```python
from build123d import *

# Parameters (mm, degrees)
F1_DEPTH = 76.2
F3_ANGLE = 90
F4_DEPTH = 203.2


with BuildPart() as f1:
    # F0 (on Front) → F1 (new body)
    with BuildSketch(Plane.XZ):
        Polygon((-6.5709403187, 0), (-3.175, -5.2222484378), (3.175, -5.2222484378), (6.7875643598, 0), (3.175, 5.2222484378), (-3.175, 5.2222484378), align=None)
    extrude(amount=F1_DEPTH)

    # F2 (on Front) → F3 (revolve)
    with BuildSketch(Plane.XZ):
        Polygon((-3.175, -5.2600912928), (3.175, -5.2600912928), (6.8761393004, 0), (3.175, 5.2600912928), (-3.175, 5.2600912928), (-6.7797889493, 0), align=None)
    revolve(axis=Axis((0, 0, 5.2600912928), (1, 0, 0)), revolution_arc=F3_ANGLE)

    # F4 (add): a face of the model
    f4_faces = [f1.faces().sort_by_distance(p)[0] for p in [
        (0.0270197551, 5.2600912928, 5.2600912928),
    ]]
    extrude(f4_faces, amount=F4_DEPTH)


solid = f1.part
```
Work out the finished part from the listing and answer in its coordinate system (mm). A direction names the side the tool comes from. Coordinates: 2 decimals unless noted, no trailing zeros. Write each loop counter-clockwise with the first axis right and the second up, starting at its lowest first coordinate (ties: lowest second). Pieces come first, ordered by that corner, then holes.
Q1. Each of these flat-tipped pins is pushed along its axis until it touches: pin 1 Ø7 at (x, y) = (0.5, -37) entering from -Z; pin 2 Ø1.5 at (x, z) = (-5, 157) entering from +Y; pin 3 Ø7 at (x, y) = (0.5, -51) entering from +Z. Where does it stop, or does it pass through?
Q2. A cutting plane is placed at B-B, the plane z = 184. Give the vertices of the cut face in (x, y) (3 decimals).
Q3. Which of the six approach directions +Z, -Z, +X, -X, +Y, -Y give full straight-line access (tool end or side, diameter ignored) to faces 1 (the face through (-4.95, 2.59, 105.44)), 2 (the face through (0, -38, 5.222)), 3 (the face through (5.051, 2.667, 105.438))?
Q4. A cutting plane is placed at C-C, the plane y = -60. Give the vertices of the cut face in (x, z) (3 decimals).
Q5. Find the intervals of material crossed by line 1 (Y direction, x = 1.5, z = 92.5); line 2 (Z direction, x = 0.5, y = -17); line 3 (Z direction, x = 6, y = -21), in increasing order.
Findings below:
1. pin 1: stops at z = -5.22
1. pin 2: stops at y = 8.95
1. pin 3: stops at z = 5.22
2. outline: (-6.78, 5.26) - (-3.175, 0) - (3.175, 0) - (6.876, 5.26) - (3.175, 10.52) - (-3.175, 10.52) - close
3. face 1: +Z, -X, -Y
3. face 2: +Z, +X, -X, -Y
3. face 3: +Z, +X, -Y
4. outline: (-6.571, 0) - (-3.175, -5.222) - (3.175, -5.222) - (6.788, 0) - (3.175, 5.222) - (-3.175, 5.222) - close
5. line 1: y = 0 to 10.52
5. line 2: z = -5.22 to 5.22
5. line 3: z = -1.14 to 1.14
